Source: CAD feature listing. Evaluate the final solid. Frame: model axes, mm. Coordinates: 2 decimals unless noted, no trailing zeros. Loops run counter-clockwise (first coordinate to the right, second up) from the corner with the lowest first, then second, coordinate; pieces in that order, holes last. Notation, with made-up numbers: (16, 35.25) - (37, 35.25) arc R14 cw to (37, 44.25) - close; hole circle Ø11 at (-29, 31.5). An arc over 180 degrees is marked (long way). Use CSV: the item, a comma, the result in double quotes. Start each with the question number.
```python
from build123d import *

# Parameters (mm, degrees)
RESSALTO_EXTRUS_O1_DEPTH = 8
ESBO_O2_W                = 32.3
ESBO_O2_H                = 16.047818473
CORTE_EXTRUS_O1_DEPTH    = 149.344709352
ESBO_O3_W                = 8
ESBO_O3_H                = 47.952181527
RESSALTO_EXTRUS_O2_DEPTH = 8
FURO_COM_FOLGA_DE_M81_D  = 9
FURO_COM_FOLGA_DE_M61_D  = 6.6
FILETE1_R                = 10


with BuildPart() as part:
    # Esboço1 → Ressalto-extrusão1 (new body)
    with BuildSketch(Plane(origin=(0, 0, 0), x_dir=(0, 0, -1), z_dir=(1, 0, 0))):
        Polygon((28, 74), (39.129876604, 32.462735031), (128.320508076, 0), (33.320508076, 0), (16, 10), (0, 10), (0, 74), align=None)
    extrude(amount=RESSALTO_EXTRUS_O1_DEPTH)

    # Esboço2 → Corte-extrusão1 (cut, through all)
    with BuildSketch(Plane(origin=(8, 0, 0), x_dir=(0, 0, -1), z_dir=(1, 0, 0))):
        with Locations((16.15, 65.976090763)):
            Rectangle(ESBO_O2_W, ESBO_O2_H)
    extrude(amount=-CORTE_EXTRUS_O1_DEPTH, mode=Mode.SUBTRACT)

    # Esboço3 → Ressalto-extrusão2 (add)
    with BuildSketch(Plane(origin=(8, 0, 0), x_dir=(0, 0, -1), z_dir=(1, 0, 0))):
        with Locations((-4, 33.976090763)):
            Rectangle(ESBO_O3_W, ESBO_O3_H)
    extrude(amount=-RESSALTO_EXTRUS_O2_DEPTH)

    # Furo com folga de M81 (through all)
    with Locations(Plane.ZY):
        with Locations((-4, 45.952181527), (-12, 22)):
            Hole(FURO_COM_FOLGA_DE_M81_D / 2)

    # Furo com folga de M61 (through all)
    with Locations(Plane(origin=(8, 0, 0), x_dir=(0, 0, -1), z_dir=(1, 0, 0))):
        with Locations((26.161384096, 49.952181527), (30.043669773, 35.463294133), (33.925955449, 20.974406739)):
            Hole(FURO_COM_FOLGA_DE_M61_D / 2)

    # Filete1
    filete1_edges = [part.edges().sort_by_distance(p)[0] for p in [
        (4, 32.462735031, -39.129876604),
    ]]
    fillet(filete1_edges, radius=FILETE1_R)


solid = part.part
```
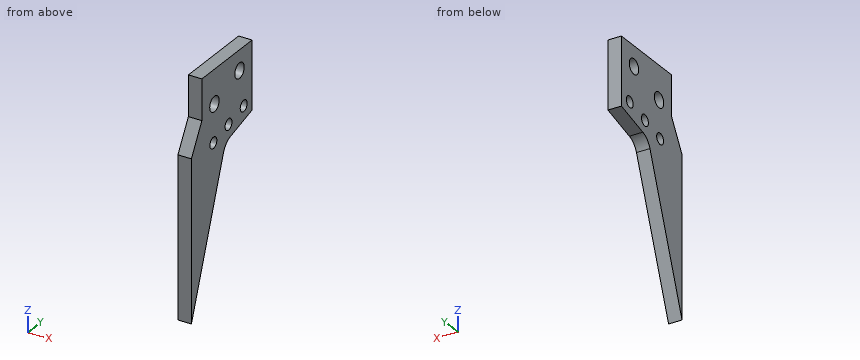
(1) Section C-C on x = 1.5. Output: boundary loops of the cut face in (y, z), plus the area to 3 significant figures.
(2) Section D-D on z = -71. Output: boundary loops of the cut face in (x, y), plus the area to 3 significant figures.
(3) Section A-A on z = -12. Output: boundary loops of the cut face in (x, y).
(4) Section B-B on y = 43.5. Output: boundary loops of the cut face in (x, z), plus the area to 3 significant figures.
(5) Ray query, line 1 (Z direction, x = 1, y = 48.5); line 2 (Y direction, x = 2.25, z = -4); line 3 (Y direction, x = 5, z = -12). Return the intervals inside material, ascending. Write a range as [from, to].
(6) Pin query (flat end, axial travel): pin 1 Ø1.5 at (x, z) = (2, -18) entering from -Y; pin 2 Ø4 at (x, z) = (3, -1.5) entering from -Y; pin 3 Ø4 at (y, z) = (35.46, -30.04) entering from +X. Return the tip coordinate at first contact, or that it passes through.
Solution:
1,outline,"(0, -128.32) - (30.68, -44.02) arc R10 cw to (37.49, -37.78) - (57.95, -32.3) - (57.95, 8) - (10, 8) - (10, -16) - (0, -33.32) - close; hole circle Ø9 at (22, -12); hole circle Ø6.6 at (20.97, -33.93); hole circle Ø6.6 at (35.46, -30.04); hole circle Ø9 at (45.95, -4); hole circle Ø6.6 at (49.95, -26.16)"
1,area,"3,540 mm²"
2,outline,"(0, 0) - (8, 0) - (8, 20.86) - (0, 20.86) - close"
2,area,"167 mm²"
3,outline,"(0, 10) - (8, 10) - (8, 17.5) - (0, 17.5) - close; (0, 26.5) - (8, 26.5) - (8, 57.95) - (0, 57.95) - close"
4,outline,"(0, -36.17) - (8, -36.17) - (8, -7.77) - (0, -7.77) - close; (0, -0.23) - (8, -0.23) - (8, 8) - (0, 8) - close"
4,area,"293 mm²"
5,line 1,"z = [-34.83, -29.12], [-23.2, -7.71], [-0.29, 8]"
5,line 2,"y = [10, 41.45], [50.45, 57.95]"
5,line 3,"y = [10, 17.5], [26.5, 57.95]"
6,pin 1,"stops at y = 8.41"
6,pin 2,"stops at y = 10"
6,pin 3,"passes through"
